```python
from build123d import *

# Parameters (mm, degrees)
F0_W     = 457.2
F0_H     = 50.8
F1_DEPTH = 9.525
F2_W     = 19.05
F2_H     = 18.4890627861
F3_DEPTH = 25.4
F4_W     = 6.35
F4_H     = 25.4
F5_DEPTH = 12.7
F6_W     = 6.35
F6_H     = 25.4
F7_DEPTH = 12.7
F8_SIZE2 = 4.478695
F8_SIZE  = 25.39999
F9_SIZE2 = 4.478695
F9_SIZE  = 25.39999


# Not quite as in the source:
# - a fillet or chamfer is up to 0.001 mm smaller than in the source, because OpenCascade refuses the exact size


with BuildPart() as f1:
    # F0 (on Right) → F1 (new body, symmetric)
    with BuildSketch(Plane.YZ):
        Rectangle(F0_W, F0_H)
    extrude(amount=F1_DEPTH, both=True)

    # F2 (on face) → F3 (cut, symmetric)
    with BuildSketch(Plane.XY.offset(25.4)):
        Rectangle(F2_W, F2_H)
    extrude(amount=F3_DEPTH, both=True, mode=Mode.SUBTRACT)

    # F4 (on face) → F5 (join, symmetric)
    with BuildSketch(Plane.XZ.offset(228.6)):
        Rectangle(F4_W, F4_H)
    extrude(amount=F5_DEPTH, both=True)

    # F6 (on face) → F7 (join, symmetric)
    with BuildSketch(Plane(origin=(0, 228.6, 0), x_dir=(-1, 0, 0), z_dir=(0, 1, 0))):
        Rectangle(F6_W, F6_H)
    extrude(amount=F7_DEPTH, both=True)

    # F8 (size 25.4 and 4.47870531 in the source; OpenCascade refuses exactly that, so slightly less here)
    f8_edges = [f1.edges().sort_by_distance(p)[0] for p in [
        (0, 241.3, -12.7),
    ]]
    f8_side = f1.faces().sort_by_distance((0, 241.3, 0))[0]
    chamfer(f8_edges, length=F8_SIZE, length2=F8_SIZE2, reference=f8_side)

    # F9 (size 25.4 and 4.47870531 in the source; OpenCascade refuses exactly that, so slightly less here)
    f9_edges = [f1.edges().sort_by_distance(p)[0] for p in [
        (0, -241.3, -12.7),
    ]]
    f9_side = f1.faces().sort_by_distance((0, -241.3, 0))[0]
    chamfer(f9_edges, length=F9_SIZE, length2=F9_SIZE2, reference=f9_side)


solid = f1.part
```
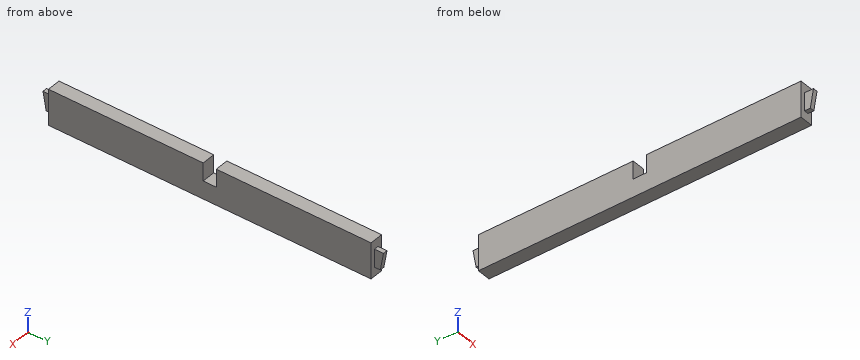
For this review, take the finished solid that the model builds, in its own axes (mm). Coordinates: 2 decimals unless noted, no trailing zeros. Loops run counter-clockwise (first coordinate to the right, second up) from the corner with the lowest first, then second, coordinate; pieces in that order, holes last. Notation, with made-up numbers: (-1.75, 77) - (35.25, 77) arc R18 ccw to (35.25, 82) - close; hole circle Ø6 at (38, 17.25). An arc over 180 degrees is marked (long way). Use one line per item in the form item = value. Start each with the question number.
1) For pin 1 (10 mm diameter, centred on y = 236, z = 2, fed in from -X) (3 decimals); pin 2 (9 mm diameter, centred on x = -4.5, y = -4, fed in from +Z); pin 3 (1.5 mm diameter, centred on x = 6.5, z = 1, fed in from +Y); pin 4 (10 mm diameter, centred on y = -232.5, z = 4, fed in from -X) (3 decimals), all flat-tipped, find the tip position at first contact; note any pin that passes through.
2) Take a section at A-A (z = 21.5). State the section outline as (x, y) points (3 decimals), plus the area to 3 significant figures.
3) Take a section at C-C (z = -7). State the section outline as (x, y) points (3 decimals), plus the area to 3 significant figures.
4) To check wall thickness, follow probe 1 along Y at (x, z) = (-8.5, 12.5); probe 2 along Y at (x, z) = (-4.5, -8); probe 3 along Y at (x, z) = (2.5, 3.5). State the ranges of each line that lie inside material, in increasing order. Write a range as from..to.
From the geometry:
q1.pin_1 = -3.175
q1.pin_2 = 0
q1.pin_3 = 228.6
q1.pin_4 = -9.525
q2.outline = (-9.525, -228.6) - (9.525, -228.6) - (9.525, -9.245) - (-9.525, -9.245) - close; (-9.525, 9.245) - (9.525, 9.245) - (9.525, 228.6) - (-9.525, 228.6) - close
q2.area = 8,360 mm2
q3.outline = (-9.525, -228.6) - (-3.175, -228.6) - (-3.175, -237.826) - (3.175, -237.826) - (3.175, -228.6) - (9.525, -228.6) - (9.525, 228.6) - (3.175, 228.6) - (3.175, 237.826) - (-3.175, 237.826) - (-3.175, 228.6) - (-9.525, 228.6) - close
q3.area = 8,830 mm2
q4.probe_1 = -228.6..-9.24, 9.24..228.6
q4.probe_2 = -228.6..228.6
q4.probe_3 = -239.68..-9.24, 9.24..239.68
